Here's how the part is built. I have some questions about the finished solid (model axes, mm). A direction names the side the tool comes from. Round coordinates to 2 decimals unless told otherwise and drop trailing zeros. Write each loop counter-clockwise with the first axis right and the second up, starting at its lowest first coordinate (ties: lowest second). Pieces come first, ordered by that corner, then holes. Notation, with made-up numbers: (83, 74) -> (90, 74) arc R18 ccw to (90, 78) -> close; hole circle Ø2 at (70, 68.25). An arc over 180 degrees is marked (long way). Answer in a Markdown table with one row per item. Add a question column.
from build123d import *

# Parameters (mm, degrees)
SKETCH1_W           = 20.25
SKETCH1_H           = 20.25
SKETCH1_R           = 9
BOSS_EXTRUDE1_DEPTH = 4.425
BOSS_EXTRUDE2_START = -1
SKETCH2_R           = 9
SKETCH2_R_2         = 7.195345153
BOSS_EXTRUDE2_DEPTH = 1
CUT_EXTRUDE1_START  = -1
CUT_EXTRUDE1_DEPTH  = 1
FILLET1_R           = 1
SKETCH4_W           = 8.85
SKETCH4_H           = 2
BOSS_EXTRUDE3_DEPTH = 1.8
CIRPATTERN1_COUNT   = 2
CIRPATTERN1_ANGLE   = 90


with BuildPart() as part:
    # Sketch1 → Boss-Extrude1 (new, symmetric)
    with BuildSketch(Plane.XY):
        Rectangle(SKETCH1_W, SKETCH1_H)
        Circle(SKETCH1_R, mode=Mode.SUBTRACT)
    extrude(amount=BOSS_EXTRUDE1_DEPTH, both=True)

    # Sketch2 → Boss-Extrude2 (add)
    with BuildSketch(Plane.XY.offset(4.425).offset(BOSS_EXTRUDE2_START)):
        Circle(SKETCH2_R)
        Circle(SKETCH2_R_2, mode=Mode.SUBTRACT)
    extrude(amount=BOSS_EXTRUDE2_DEPTH)

    # Sketch3 → Cut-Extrude1 (cut)
    with BuildSketch(Plane.XY.offset(4.425).offset(CUT_EXTRUDE1_START)):
        with BuildLine():
            Line((-10.125, -5), (-5.174262446, -5))
            ThreePointArc((-5.174262446, -5), (-5.08787735, -5.08787735), (-5, -5.174262446))
            Line((-5, -5.174262446), (-5, -10.125))
            Line((-5, -10.125), (5, -10.125))
            Line((5, -10.125), (5, -5.174262446))
            ThreePointArc((5, -5.174262446), (5.08787735, -5.08787735), (5.174262446, -5))
            Line((5.174262446, -5), (10.125, -5))
            Line((10.125, -5), (10.125, 5))
            Line((10.125, 5), (5.174262446, 5))
            ThreePointArc((5.174262446, 5), (5.08787735, 5.08787735), (5, 5.174262446))
            Line((5, 5.174262446), (5, 10.125))
            Line((5, 10.125), (-5, 10.125))
            Line((-5, 10.125), (-5, 5.174262446))
            ThreePointArc((-5, 5.174262446), (-5.08787735, 5.08787735), (-5.174262446, 5))
            Line((-5.174262446, 5), (-10.125, 5))
            Line((-10.125, 5), (-10.125, -5))
        make_face()
    extrude(amount=CUT_EXTRUDE1_DEPTH, mode=Mode.SUBTRACT)

    # Fillet1
    fillet1_edges = [part.edges().sort_by_distance(p)[0] for p in [
        (-10.125, 10.125, 0),
        (10.125, 10.125, 0),
        (10.125, -10.125, 0),
        (-10.125, -10.125, 0),
    ]]
    fillet(fillet1_edges, radius=FILLET1_R)

    # Sketch4 → Boss-Extrude3 (add)
    with BuildSketch(Plane.ZY.offset(10.125)):
        with Locations((0, 7)):
            Rectangle(SKETCH4_W, SKETCH4_H)
        with Locations((0, -7)):
            Rectangle(SKETCH4_W, SKETCH4_H)
    boss_extrude3 = extrude(amount=BOSS_EXTRUDE3_DEPTH)

    # CirPattern1: Boss-Extrude3 ×2 about axis
    cirpattern1_axis = Axis((0, 0, 0), (0, 0, -1))
    for i in range(1, CIRPATTERN1_COUNT):
        add(boss_extrude3.rotate(cirpattern1_axis, i * CIRPATTERN1_ANGLE / (CIRPATTERN1_COUNT - 1)))


solid = part.part
Item 1: If we section it at A-A on x = 0: Please give me the cut outline in (y, z) (3 decimals).
Item 2: If we section it at B-B on z = -1: Please give me the cut outline in (x, y) (3 decimals), then the cut area to 3 significant figures.
Item 3: I need wall thicknesses on line 1 along Y through (x, z) = (0, -1) (3 decimals); line 2 along X through (y, z) = (10.5, 1.25); line 3 along Z through (x, y) = (4.5, -9) (3 decimals). Which ranges of each line are inside material? Lowest first, please. Write a range as from..to.
Item 4: If we mould it in two halves opening along Y, with no side actions, what happens to faces 1 (the flat face through (0, 10.125, 0)), 2 (the flat face through (-6, 6, 3.425)), 3 (the flat face through (-6, 11, 0))? For each: pulls with the +Y half, pulls with the -Y half, needs draft (parallel to the pull), parting line crosses it, or undercut.
Item 5: On a 3-axis mill with a long thin cutter (end or side, diameter ignored), from which of +Z, -Z, +X, -X, +Y, -Y can I reach the whole of each face in a straight line? I mean faces 4 (the flat face through (6, 11, 0)), 5 (the flat face through (-11, 6, 0)), 6 (the flat face through (-11, 8, 0)), 7 (the cylindrical face through (-1.172, 8.923, -0.555)). Say none if no direction works.
Item 6: For P1, Ø0.8, axis at x = -8.5, y = -1.5, coming from the +Z side (3 decimals); P2, Ø2.5, axis at y = -1.5, z = 1, coming from the -X side (3 decimals); P3, Ø1.5, axis at x = 2.5, z = -1, coming from the +Y side (3 decimals), each with a flat end and sliding along its axis, tell me the tip position at first contact or that it passes through.
Results list:
| question | item | result |
|---|---|---|
| 1 | outline | (-10.125, -4.425) -> (-9, -4.425) -> (-9, 3.425) -> (-10.125, 3.425) -> close; (9, -4.425) -> (10.125, -4.425) -> (10.125, 3.425) -> (9, 3.425) -> close |
| 2 | outline | (-11.925, -8) -> (-10.125, -8) -> (-10.125, -9.125) arc R1 ccw to (-9.125, -10.125) -> (9.125, -10.125) arc R1 ccw to (10.125, -9.125) -> (10.125, 9.125) arc R1 ccw to (9.125, 10.125) -> (8, 10.125) -> (8, 11.925) -> (6, 11.925) -> (6, 10.125) -> (-6, 10.125) -> (-6, 11.925) -> (-8, 11.925) -> (-8, 10.125) -> (-9.125, 10.125) arc R1 ccw to (-10.125, 9.125) -> (-10.125, 8) -> (-11.925, 8) -> (-11.925, 6) -> (-10.125, 6) -> (-10.125, -6) -> (-11.925, -6) -> close; hole circle Ø18 at (0, 0) |
| 2 | area | 169 mm² |
| 3 | line 1 | -10.125..-9, 9..10.125 |
| 3 | line 2 | -8..-6, 6..8 |
| 3 | line 3 | -4.425..3.425 |
| 4 | face 1 | pulls with the +Y half |
| 4 | face 2 | undercut |
| 4 | face 3 | needs draft |
| 5 | face 4 | +Z, -Z, +Y |
| 5 | face 5 | +Z, -Z, -X |
| 5 | face 6 | +Z, -Z, -X, +Y |
| 5 | face 7 | -Z |
| 6 | P1 | z = 3.425 |
| 6 | P2 | x = -10.125 |
| 6 | P3 | y = 10.125 |
